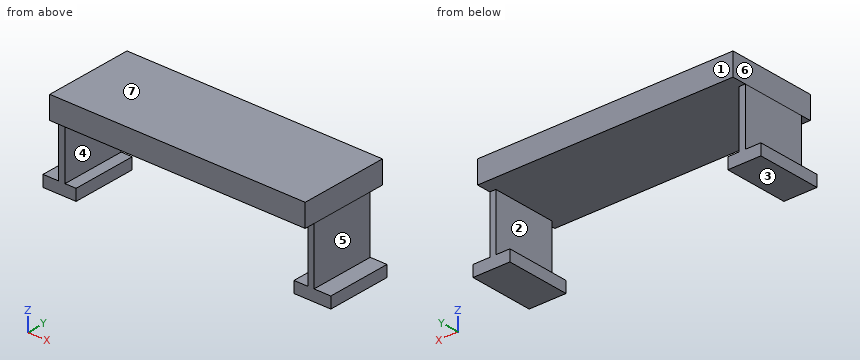
```python
from build123d import *

# Parameters (mm, degrees)
F0_W     = 112.853165
F0_H     = 39.353924
F1_DEPTH = 10
F2_W     = 2.840738
F2_H     = 28.620001
F2_W_2   = 2.645086
F3_DEPTH = 25
F4_W     = 14.609244
F4_H     = 28.620001
F5_DEPTH = 5
F6_W     = 16.285717
F6_H     = 28.620001
F7_DEPTH = 5


with BuildPart() as f1:
    # F0 (on Top) → F1 (new body)
    with BuildSketch(Plane.XY):
        with Locations((1.59152, -0.578734)):
            Rectangle(F0_W, F0_H)
    extrude(amount=F1_DEPTH)

    # F2 (on face) → F3 (join)
    with BuildSketch(Plane(origin=(0, 0, 0), x_dir=(1, 0, 0), z_dir=(0, 0, -1))):
        with Locations((-53.414693, 1.450803)):
            Rectangle(F2_W, F2_H)
        with Locations((56.69556, 1.450803)):
            Rectangle(F2_W_2, F2_H)
    extrude(amount=F3_DEPTH)

    # F4 (on face) → F5 (join)
    with BuildSketch(Plane(origin=(0, 0, -25), x_dir=(1, 0, 0), z_dir=(0, 0, -1))):
        with Locations((-54.408634, 1.450803)):
            Rectangle(F4_W, F4_H)
    extrude(amount=F5_DEPTH)

    # F6 (on face) → F7 (join)
    with BuildSketch(Plane(origin=(0, 0, -25), x_dir=(1, 0, 0), z_dir=(0, 0, -1))):
        with Locations((57.296015, 1.450803)):
            Rectangle(F6_W, F6_H)
    extrude(amount=F7_DEPTH)


solid = f1.part
```
Can you work these out from the model? Positions are in its coordinate system, mm. Face numbers are marked on the shaded views. A direction names the side the tool comes from. Coordinates: 2 decimals unless noted, no trailing zeros. Order: outer loops, then holes, each group sorted by start corner. A loop starts at its lowest first (then second) coordinate and runs counter-clockwise, first axis right, second up. Notation, with made-up numbers: (38, -23.5) - (77, -23.5) arc R18 ccw to (77, -2.5) - close; hole circle Ø8 at (21, 30.25). An arc over 180 degrees is marked (long way). Answer in a Markdown table with one row per item.
1. If we mould it in two halves opening along Z, with no side actions, what happens to the marked faces 1, 2 and 3? For each: pulls with the +Z half, pulls with the -Z half, needs draft (parallel to the pull), parting line crosses it, or undercut.
Reply:
| item | result |
|---|---|
| face 1 | needs draft |
| face 2 | undercut |
| face 3 | pulls with the -Z half |
2. For the marked faces 4, 5, 6 and 7, which set-ups out of +Z, -Z, +X, -X, +Y, -Y let a thin tool reach every point of the face, with its end or its side?
Reply:
| item | result |
|---|---|
| face 4 | +Y, -Y |
| face 5 | +Z, +X, +Y, -Y |
| face 6 | +Z, -X, +Y, -Y |
| face 7 | +Z, +X, -X, +Y, -Y |
3. If I drill on line 1 along X through (y, z) = (0, -12); line 2 along Z through (x, y) = (-51, -5); line 3 along Z through (x, y) = (40, 4), over which ranges is the centre line in solid material (lowest first)?
Reply:
| item | result |
|---|---|
| line 1 | x = -54.84 to -51.99, 55.37 to 58.02 |
| line 2 | z = -30 to -25, 0 to 10 |
| line 3 | z = 0 to 10 |
4. Suppose I cut it at B-B (x = 53). Please give me the cut outline in (y, z), and give its area (3 significant figures).
Reply:
| item | result |
|---|---|
| outline | (-20.26, 0) - (19.1, 0) - (19.1, 10) - (-20.26, 10) - close; (-15.76, -30) - (12.86, -30) - (12.86, -25) - (-15.76, -25) - close |
| area | 537 mm^2 |
5. Suppose I cut it at C-C (y = -10). Please give me the cut outline in (x, z), and give its area (3 significant figures).
Reply:
| item | result |
|---|---|
| outline | (-61.71, -30) - (-47.1, -30) - (-47.1, -25) - (-51.99, -25) - (-51.99, 0) - (55.37, 0) - (55.37, -25) - (49.15, -25) - (49.15, -30) - (65.44, -30) - (65.44, -25) - (58.02, -25) - (58.02, 10) - (-54.84, 10) - (-54.84, -25) - (-61.71, -25) - close |
| area | 1,420 mm^2 |
6. Suppose I cut it at D-D (x = -35.5). Please give me the cut outline in (y, z).
Reply:
| item | result |
|---|---|
| outline | (-20.26, 0) - (19.1, 0) - (19.1, 10) - (-20.26, 10) - close |
7. Suppose I cut it at A-A (z = -19). Please give me the cut outline in (x, y).
Reply:
| item | result |
|---|---|
| outline | (-54.84, -15.76) - (-51.99, -15.76) - (-51.99, 12.86) - (-54.84, 12.86) - close; (55.37, -15.76) - (58.02, -15.76) - (58.02, 12.86) - (55.37, 12.86) - close |
8. For pin 1 (3 mm diameter, centred on y = 3, z = -14, fed in from +X); pin 2 (5 mm diameter, centred on y = 6, z = 3, fed in from -X); pin 3 (11.5 mm diameter, centred on x = -51, z = -18.5, fed in from -Y), each with a flat end and sliding along its axis, tell me the tip position at first contact or that it passes through.
Reply:
| item | result |
|---|---|
| pin 1 | stops at x = 58.02 |
| pin 2 | stops at x = -54.84 |
| pin 3 | stops at y = -15.76 |
